Design review of the part built by this model. Coordinates are the model's own, in mm. Coordinates: 2 decimals unless noted, no trailing zeros. Order: outer loops, then holes, each group sorted by start corner. A loop starts at its lowest first (then second) coordinate and runs counter-clockwise, first axis right, second up. Notation, with made-up numbers: (72, 21) -> (117, 21) arc R25 ccw to (117, 51) -> close; hole circle Ø10 at (-17, 89). An arc over 180 degrees is marked (long way). Write item = value, one per line.
```python
from build123d import *

# Parameters (mm, degrees)
F0_W           = 63.1470456719
F0_H           = 44.8482893407
F1_DEPTH       = 25
F3_D           = 7.1374
F3_CSINK_D     = 13.4874
F3_CSINK_ANGLE = 82
F4_R           = 5


with BuildPart() as f1:
    # F0 (on Front) → F1 (new body)
    with BuildSketch(Plane.XZ):
        with Locations((31.573522836, -22.4241446704)):
            Rectangle(F0_W, F0_H)
    extrude(amount=F1_DEPTH)

    # F3 (through all)
    with Locations(Plane.XZ.offset(25)):
        with Locations((29.9805495888, -23.4452802688)):
            CounterSinkHole(F3_D / 2, F3_CSINK_D / 2, counter_sink_angle=F3_CSINK_ANGLE)

    # F4
    f4_edges = [f1.edges().sort_by_distance(p)[0] for p in [
        (63.147046, -12.5, 0),
        (0, -12.5, 0),
        (31.573523, 0, 0),
        (31.573523, -25, 0),
        (0, -12.5, -44.848289),
        (0, 0, -22.424145),
        (0, -25, -22.424145),
        (63.147046, -12.5, -44.848289),
        (31.573523, 0, -44.848289),
        (31.573523, -25, -44.848289),
        (63.147046, 0, -22.424145),
        (63.147046, -25, -22.424145),
    ]]
    fillet(f4_edges, radius=F4_R)


solid = f1.part
```
(1) We need section A-A (y = -12). Write out the cut boundary in (x, z).
Report:
outline = (0, -39.85) arc R5 ccw to (5, -44.85) -> (58.15, -44.85) arc R5 ccw to (63.15, -39.85) -> (63.15, -5) arc R5 ccw to (58.15, 0) -> (5, 0) arc R5 ccw to (0, -5) -> close; hole circle Ø7.14 at (29.98, -23.45)
(2) Insertion check: pin 1 (4.5 mm diameter, centred on x = 29.98, z = -23.45, fed in from +Y). The pin has a flat end and moves straight along its axis. Give the tip position at first contact, or say it passes through.
Report:
pin_1 = through
(3) We need section C-C (x = 55.5). Write out the cut boundary in (y, z).
Report:
outline = (-25, -39.85) arc R5 ccw to (-20, -44.85) -> (-5, -44.85) arc R5 ccw to (0, -39.85) -> (0, -5) arc R5 ccw to (-5, 0) -> (-20, 0) arc R5 ccw to (-25, -5) -> close
(4) The part is to be moulded in two halves that separate along Z. For faces 1 (the flat face through (0, -12, -23)), 2 (the cylindrical face through (26.684, -10.524, -24.812)), 3 (the cylindrical face through (61.721, -12.605, -43.345)), say which applies: released by +Z, released by -Z, zero draft, split by the parting line, or undercut.
Report:
face_1 = zero draft
face_2 = undercut
face_3 = released by -Z
(5) For L1, parallel to X at y = -9.5, z = -22; L2, parallel to X at y = -1.75, z = -22; L3, parallel to Z at x = 29, y = -19.5, list the stretches that pass through material, from the lowest coordinate up.
Report:
L1 = 0 to 26.72, 33.24 to 63.15
L2 = 1.2 to 26.72, 33.24 to 61.95
L3 = -44.85 to -26.88, -20.01 to 0
(6) We need section B-B (z = -4). Write out the cut boundary in (x, y), and give its area (3 significant figures).
Report:
outline = (0.1, -20) arc R4.9 ccw to (5, -24.9) -> (58.15, -24.9) arc R4.9 ccw to (63.05, -20) -> (63.05, -5) arc R4.9 ccw to (58.15, -0.1) -> (5, -0.1) arc R4.9 ccw to (0.1, -5) -> close
area = 1,540 mm²
